```python
from build123d import *

# Parameters (mm, degrees)
SKETCH_1_R      = 25
SKETCH_1_R_2    = 12.5
SKETCH_1_R_3    = 4
EXTRUDE_1_DEPTH = 6
SKETCH_1_3_R    = 12.5
SKETCH_1_3_R_2  = 4
EXTRUDE_2_DEPTH = 10


with BuildPart() as part:
    # Sketch 1 → Extrude 1 (new body)
    with BuildSketch(Plane.XY):
        Circle(SKETCH_1_R)
        Circle(SKETCH_1_R_2, mode=Mode.SUBTRACT)
        Circle(SKETCH_1_R_2)
        Circle(SKETCH_1_R_3, mode=Mode.SUBTRACT)
    extrude(amount=EXTRUDE_1_DEPTH)

    # Sketch 1_3 → Extrude 2 (add)
    with BuildSketch(Plane.XY):
        Circle(SKETCH_1_3_R)
        Circle(SKETCH_1_3_R_2, mode=Mode.SUBTRACT)
    extrude(amount=-EXTRUDE_2_DEPTH)


solid = part.part
```
Design review of the part built by this model. Coordinates are the model's own, in mm. A direction names the side the tool comes from. Coordinates: 2 decimals unless noted, no trailing zeros. Order: outer loops, then holes, each group sorted by start corner. A loop starts at its lowest first (then second) coordinate and runs counter-clockwise, first axis right, second up. Notation, with made-up numbers: (-16, 26.5) -> (-1, 26.5) arc R28 ccw to (-1, 56.5) -> close; hole circle Ø3 at (-3, -17.5). An arc over 180 degrees is marked (long way). One line per item, written item: value. Start each with the question number.
Q1. Take a section at D-D, the plane y = -15.5. State the section outline as (x, z) points, then the cut area to 3 significant figures.
Q2. Take a section at C-C, the plane z = -7.75. State the section outline as (x, y) points.
Q3. For probe 1 along Y at (x, z) = (0, 2.7); probe 2 along Y at (x, z) = (0, -7); probe 3 along Z at (x, y) = (-11, 21.5), list the stretches that pass through material, from the lowest coordinate up.
Q4. Take a section at A-A, the plane y = 0. State the section outline as (x, z) points.
Q5. Tool access review of faces 1 (the flat face through (-3, 3, -10)), 2 (the cylindrical face through (11.923, 3.755, -4.93)): name each direction out of +Z, -Z, +X, -X, +Y, -Y from which nothing blocks a thin tool from reaching the whole face with its end or side.
Q6. Insertion check: pin 1 Ø12 at (x, y) = (19, -8.5) entering from -Z; pin 2 Ø4 at (x, z) = (4.5, 3.5) entering from -Y; pin 3 Ø5 at (x, z) = (-8, 0) entering from +Y. Each pin has a flat end and moves straight along its axis. Give the tip position at first contact, or say it passes through.
Values follow:
1. outline: (-19.62, 0) -> (19.62, 0) -> (19.62, 6) -> (-19.62, 6) -> close
1. area: 235 mm2
2. outline: circle Ø25 at (0, 0); hole circle Ø8 at (0, 0)
3. probe 1: y = -25 to -4, 4 to 25
3. probe 2: y = -12.5 to -4, 4 to 12.5
3. probe 3: z = 0 to 6
4. outline: (-25, 0) -> (-12.5, 0) -> (-12.5, -10) -> (-4, -10) -> (-4, 6) -> (-25, 6) -> close; (4, -10) -> (12.5, -10) -> (12.5, 0) -> (25, 0) -> (25, 6) -> (4, 6) -> close
5. face 1: -Z, +X, -X, +Y, -Y
5. face 2: -Z
6. pin 1: stops at z = 0
6. pin 2: stops at y = -24.87
6. pin 3: stops at y = 24.39
